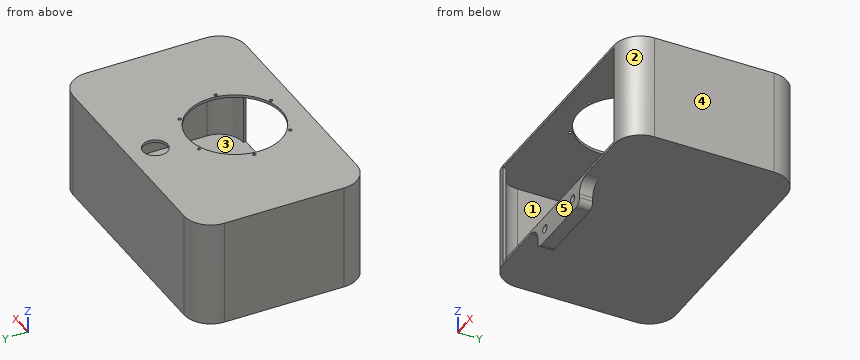
```python
from build123d import *

# Parameters (mm, degrees)
BOSS_EXTRU_1_DEPTH      = 40
COQUE1_START            = 1
COQUE1_DEPTH            = 38
ESQUISSE2_R             = 4.67
ESQUISSE2_R_2           = 17.660377339
ESQUISSE2_R_3           = 0.603773585
ESQUISSE2_R_4           = 0.543253327
ENL_V_MAT_EXTRU_1_DEPTH = 5
ESQUISSE3_R             = 1.5
BOSS_EXTRU_2_DEPTH      = 5
CONG_1_R                = 5


# Read off the part's stored shape, not the designer's step: Coque1
with BuildPart() as part:
    # Esquisse1 → Boss.-Extru.1 (new body)
    with BuildSketch(Plane.XY):
        with BuildLine():
            Line((-40, 32.5), (40, 32.5))
            ThreePointArc((40, 32.5), (47.071067812, 29.571067812), (50, 22.5))
            Line((50, 22.5), (50, -22.5))
            ThreePointArc((50, -22.5), (47.071067812, -29.571067812), (40, -32.5))
            Line((40, -32.5), (-40, -32.5))
            ThreePointArc((-40, -32.5), (-47.071067812, -29.571067812), (-50, -22.5))
            Line((-50, -22.5), (-50, 22.5))
            ThreePointArc((-50, 22.5), (-47.071067812, 29.571067812), (-40, 32.5))
        make_face()
    extrude(amount=BOSS_EXTRU_1_DEPTH)

    # Coque1 outline → Coque1 (cut)
    with BuildSketch(Plane.XY.offset(COQUE1_START)):
        with BuildLine():
            Line((-40, -31.5), (-40, -32.5))
            Line((-40, -32.5), (40, -32.5))
            Line((40, -32.5), (40, -31.5))
            ThreePointArc((40, -31.5), (46.363961031, -28.863961031), (49, -22.5))
            Line((49, -22.5), (49, 22.5))
            ThreePointArc((49, 22.5), (46.363961031, 28.863961031), (40, 31.5))
            Line((40, 31.5), (-40, 31.5))
            ThreePointArc((-40, 31.5), (-46.363961031, 28.863961031), (-49, 22.5))
            Line((-49, 22.5), (-49, -22.5))
            ThreePointArc((-49, -22.5), (-46.363961031, -28.863961031), (-40, -31.5))
        make_face()
    extrude(amount=COQUE1_DEPTH, mode=Mode.SUBTRACT)

    # Esquisse2 → Enlèv. mat.-Extru.1 (cut)
    with BuildSketch(Plane.XY.offset(40)):
        with Locations((0.168563894, 22.39389783)):
            Circle(ESQUISSE2_R)
        with Locations((-2.4e-08, -7.499999903)):
            Circle(ESQUISSE2_R_2)
        with Locations((-18.557820098, -5.064287395)):
            Circle(ESQUISSE2_R_3)
        with Locations((18.557820098, -9.935712605)):
            Circle(ESQUISSE2_R_3)
        with Locations((11.388299042, 7.353687341)):
            Circle(ESQUISSE2_R_3)
        with Locations((-7.169521057, 9.789399947)):
            Circle(ESQUISSE2_R_4)
        with Locations((7.169521057, -24.789399947)):
            Circle(ESQUISSE2_R_3)
        with Locations((-11.388299042, -22.353687341)):
            Circle(ESQUISSE2_R_3)
    extrude(amount=-ENL_V_MAT_EXTRU_1_DEPTH, mode=Mode.SUBTRACT)

    # Esquisse3 → Boss.-Extru.2 (add)
    with BuildSketch(Plane.XZ.offset(32.5)):
        with BuildLine():
            Line((-12.5, -9), (12.5, -9))
            ThreePointArc((12.5, -9), (14.267766953, -8.267766953), (15, -6.5))
            Line((15, -6.5), (15, 1))
            Line((15, 1), (-15, 1))
            Line((-15, 1), (-15, -6.5))
            ThreePointArc((-15, -6.5), (-14.267766953, -8.267766953), (-12.5, -9))
        make_face()
        with Locations(Location((-10, -4, 0), (0, 0, 270))):
            Circle(ESQUISSE3_R, mode=Mode.SUBTRACT)
        with Locations(Location((10, -4, 0), (0, 0, 90))):
            Circle(ESQUISSE3_R, mode=Mode.SUBTRACT)
    extrude(amount=-BOSS_EXTRU_2_DEPTH)

    # Congé1
    cong_1_edges = [part.edges().sort_by_distance(p)[0] for p in [
        (-15, -30, 0),
        (15, -30, 0),
    ]]
    fillet(cong_1_edges, radius=CONG_1_R)


solid = part.part
```
Geometry: final body of the model. Coordinates: model frame, mm. Face numbers are marked on the shaded views. A direction names the side the tool comes from. Round coordinates to 2 decimals unless told otherwise and drop trailing zeros. Order: outer loops, then holes, each group sorted by start corner. A loop starts at its lowest first (then second) coordinate and runs counter-clockwise, first axis right, second up. Notation, with made-up numbers: M -21.75,84 L 26.25,84 A29 ccw 26.25,111 Z; hole C 6.25,2.5 d7. An arc over 180 degrees is marked long. Use one line per item in the form item = value. Start each with the question number.
Q1. Pin query (flat end, axial travel): pin 1 Ø1 at (x, y) = (-11.39, -22.35) entering from +Z; pin 2 Ø12 at (x, y) = (-9.5, -2) entering from -Z; pin 3 Ø5 at (x, z) = (10, -4) entering from +Y. Return the tip coordinate at first contact, or that it passes through.
Q2. Cut plane C-C (y = -7.5). Return loops of the section in (x, z).
Q3. Mould query, pull axis Y, two halves, no side actions, for the marked faces 3, 4 and 5. Classes: +Y half, -Y half, draft (parallel to the pull), parting line (faces both ways), or undercut.
Q4. Cut plane D-D (y = 28.5). Return loops of the section in (x, z).
Q5. Material intervals for line 1 (Z direction, x = -16, y = -27); line 2 (X direction, y = 10, z = 15.5); line 3 (X direction, y = -31, z = -4), sorted ascending. Write a range as [from, to].
Q6. Cut plane B-B (x = 35.5). Return loops of the section in (y, z).
Q7. Cut plane A-A (z = 3). Return loops of the section in (x, y), and give its area (3 significant figures).
Q8. Access query for the marked faces 1 and 2. Directions: +Z, -Z, +X, -X, +Y, -Y. A direction counts if a zero-diameter tool reaches every point of the face in a straight line with its end or side. Return the directions, or none.
Geometry results:
q1.pin_1 = 1
q1.pin_2 = 0
q1.pin_3 = -27.5
q2.outline = M -50,0 L 50,0 L 50,40 L 17.66,40 L 17.66,39 L 49,39 L 49,1 L -49,1 L -49,39 L -17.66,39 L -17.66,40 L -50,40 Z
q3.face_3 = undercut
q3.face_4 = draft
q3.face_5 = -Y half
q4.outline = M -48,0 L 48,0 L 48,40 L -48,40 Z; hole M -46.71,1 L 46.71,1 L 46.71,39 L -46.71,39 Z
q5.line_1 = [0, 1], [39, 40]
q5.line_2 = [-50, -49], [49, 50]
q5.line_3 = [-15.1, -11.5], [-8.5, 8.5], [11.5, 15.1]
q6.outline = M -32.5,0 L 32.5,0 L 32.5,40 L -32.5,40 L -32.5,39 L 31.5,39 L 31.5,1 L -32.5,1 Z
q7.outline = M -50,-22.5 A10 ccw -40,-32.5 L -40,-31.5 A9 cw -49,-22.5 L -49,22.5 A9 cw -40,31.5 L 40,31.5 A9 cw 49,22.5 L 49,-22.5 A9 cw 40,-31.5 L 40,-32.5 A10 ccw 50,-22.5 L 50,22.5 A10 ccw 40,32.5 L -40,32.5 A10 ccw -50,22.5 Z
q7.area = 230 mm^2
q8.face_1 = none
q8.face_2 = +Z, -Z, +X, -Y
